```python
from build123d import *

# Parameters (mm, degrees)
SKETCH1_W   = 16.0655
SKETCH1_H   = 52.07
SKETCH1_W_2 = 2.450561434
SKETCH1_H_2 = 35.306


with BuildPart() as part:
    # Sketch1 → Revolve1 (revolve)
    with BuildSketch(Plane.XY, mode=Mode.PRIVATE) as revolve1_sk:
        with Locations((8.03275, -26.035)):
            Rectangle(SKETCH1_W, SKETCH1_H)
        with Locations((1.225280717, 17.653)):
            Rectangle(SKETCH1_W_2, SKETCH1_H_2)
        Polygon((0, 37.846), (0, 35.306), (2.450561434, 35.306), (14.836359841, 35.306), (14.836359841, 37.846), align=None)
    revolve(revolve1_sk.sketch.rotate(Axis((0, 0, 0), (0, 1, 0)), 90), axis=Axis((0, 0, 0), (0, 1, 0)))


solid = part.part
```
Read the model definition and answer for the solid it produces. Units are mm, in the model's axes. A direction names the side the tool comes from. Coordinates: 2 decimals unless noted, no trailing zeros. Order: outer loops, then holes, each group sorted by start corner. A loop starts at its lowest first (then second) coordinate and runs counter-clockwise, first axis right, second up. Notation, with made-up numbers: (-7.75, 73.25) - (30.25, 73.25) arc R21 ccw to (30.25, 79.25) - close; hole circle Ø9 at (22, 47). An arc over 180 degrees is marked (long way). Answer as a JSON object with one key per item and string values. Group by question number.
Item 1: Flat-ended cylindrical pins translate along their axes: P1, Ø10, axis at x = 9, y = -15, coming from the +Z side; P2, Ø10, axis at x = 2, y = 26, coming from the -Z side; P3, Ø6, axis at x = -6, y = -2.5, coming from the -Z side. Find the tip coordinate at first contact, or state that the pin passes through.
Item 2: Section C-C (x = -7.5) is taken. Give the vertices of the cut face in (y, z).
Item 3: Section D-D (y = 11) is taken. Give the vertices of the cut face in (x, z).
Item 4: A tool of negligible diameter and unlimited length cuts with its end or side. For faces 1 (the face through (2.174, 17.9, -1.131)), 2 (the face through (0, -52.07, 0)), 3 (the face through (-14.71, 36.59, 1.93)), from which of +Z, -Z, +X, -X, +Y, -Y can it reach the whole face along a straight path? Write none if from no direction.
Item 5: Section A-A (z = -7.5) is taken. Give the vertices of the cut face in (x, y), plus the area to 3 significant figures.
Item 6: Consider probe 1 along Y at (x, z) = (0, 5); probe 2 along Y at (x, z) = (14.5, -6); probe 3 along X at (y, z) = (-44.5, 10.5). Determine where each line is inside the solid, lowest interval first. Write a range as from..to.
Item 7: Section B-B (x = 0) is taken. Give the vertices of the cut face in (y, z), plus the area to 3 significant figures.
Results are:
{
 "1": {"P1": "stops at z = 15.56", "P2": "stops at z = -2.45", "P3": "stops at z = -15.78"},
 "2": {"outline": "(-52.07, -14.21) - (0, -14.21) - (0, 14.21) - (-52.07, 14.21) - close; (35.31, -12.8) - (37.85, -12.8) - (37.85, 12.8) - (35.31, 12.8) - close"},
 "3": {"outline": "circle Ø4.9 at (0, 0)"},
 "4": {"face 1": "none", "face 2": "+Z, -Z, +X, -X, -Y", "face 3": "+Y"},
 "5": {"outline": "(-14.21, -52.07) - (14.21, -52.07) - (14.21, 0) - (-14.21, 0) - close; (-12.8, 35.31) - (12.8, 35.31) - (12.8, 37.85) - (-12.8, 37.85) - close", "area": "1,540 mm^2"},
 "6": {"probe 1": "y = -52.07..0, 35.31..37.85", "probe 2": "y = -52.07..0", "probe 3": "x = -12.16..12.16"},
 "7": {"outline": "(-52.07, -16.07) - (0, -16.07) - (0, -2.45) - (35.31, -2.45) - (35.31, -14.84) - (37.85, -14.84) - (37.85, 14.84) - (35.31, 14.84) - (35.31, 2.45) - (0, 2.45) - (0, 16.07) - (-52.07, 16.07) - close", "area": "1,920 mm^2"}
}
